Autodesk Inventor part; units mm, degrees
ref_plane "YZ Plane" through (0, 0, 0) normal (1, 0, 0) x (0, 1, 0)
ref_plane "XZ Plane" through (0, 0, 0) normal (0, 1, 0) x (-1, 0, 0)
ref_plane "XY Plane" through (0, 0, 0) normal (0, 0, 1) x (1, 0, 0)
sketch "Skizze1" plane through (0, 0, 0) normal (0, 1, 0) x (-1, 0, 0)
  line L0 (0, 25) -> (0, -25)
  line L1 (0, -25) -> (8, -25)
  line L2 (8, -25) -> (67.4432, -9.1805)
  arc A0 (67.4432, -9.1805) -> (67.4432, 9.1805) centre (65, 0) ccw
  line L3 (67.4432, 9.1805) -> (8, 25)
  line L4 (8, 25) -> (0, 25)
  line L5 (0, 0) -> (65, 0) construction
  dimension "d0" = 9.5
  dimension "d1" = 50
  dimension "d2" = 8
  dimension "d3" = 65
extrude "Extrusion1" add sketch "Skizze1" along normal blind 2
sketch "Skizze2" plane through (0, 2, 0) normal (0, 1, 0) x (1, 0, 0)
  line L0 (-67.4432, -9.1805) -> (-8, -25)
  line L1 (0, 25) -> (-8, 25)
  line L2 (-8, -25) -> (0, -25)
  line L3 (0, -25) -> (0, 25)
  line L4 (0, 25) -> (-8, 25)
  line L5 (-8, 25) -> (-8, -25)
  point P0 (0, 0)
  point P1 (-8, 25)
extrude "Extrusion2" add sketch "Skizze2" along normal blind 6.5
sketch "Skizze3" plane through (-8, 2, -25) normal (-1, 0, 0) x (0, 0, 1)
  line L0 (50, -2) -> (0, -2)
  line L1 (0, 6.5) -> (50, 6.5)
  line L2 (25, 6.5) -> (25, -12.2708) construction
  point P0 (25, -2)
  point P1 (46.124, 3)
  point P2 (3.876, 3)
  dimension "d15" = 5
  dimension "d33" = 42.248
hole "Bohrung1" at (-8, 5, 21.124) at (-8, 5, -21.124) direction (1, 0, 0) diameter 5 depth 8
sketch "Skizze4" plane through (0, 2, 0) normal (0, 1, 0) x (1, 0, 0)
  arc A0 (-67.4432, 9.1805) -> (-67.4432, -9.1805) centre (-65, 0) ccw
  point P0 (0, 0)
hole "Bohrung2" at (-65, 2, 0) direction (0, -1, 0) diameter 10 depth 2
sketch "Skizze5" plane through (0, 2, 0) normal (0, 1, 0) x (1, 0, 0)
  arc A0 (-67.4432, 9.1805) -> (-67.4432, -9.1805) centre (-65, 0) ccw
  point P0 (0, 0)
  point P1 (-51.97, 0)
  point P2 (-74.5, 0)
  dimension "d32" = 13.03
hole "Bohrung3" at (-51.97, 2, 0) direction (0, -1, 0) diameter 3.5 depth 2
properties part number "05" material "Aluminium 6061"
Build history of the part. All positions in model axes, mm. A direction names the side the tool comes from. Round coordinates to 2 decimals unless told otherwise and drop trailing zeros. Write each loop counter-clockwise with the first axis right and the second up, starting at its lowest first coordinate (ties: lowest second). Pieces come first, ordered by that corner, then holes.
1) Band-saw the part on B-B, the plane y = 5. List the corners of the cut face in (x, z), and give its area (3 significant figures).
2) Band-saw the part on D-D, the plane z = 22. List the corners of the cut face in (x, y).
3) Drill centre lines: probe 1 along X at (y, z) = (1.25, 0); probe 2 along Z at (x, y) = (-4.75, 5); probe 3 along Y at (x, z) = (-41.5, -2). Where is each one in solid material? Low to high.
4) Pin check, flat tips, straight feed: pin 1 (1 mm diameter, centred on x = -42.5, z = 3.5, fed in from -Y); pin 2 (1.5 mm diameter, centred on y = 6.5, z = -15.5, fed in from -X); pin 3 (16 mm diameter, centred on x = -65, z = 0, fed in from +Y). Stop position of each tip, or through.
5) Band-saw the part on C-C, the plane x = -65. List the corners of the cut face in (y, z), and give its area (3 significant figures).
6) Mould opens along Z. For faces 1 (the cylindrical face through (-3.94, 4.25, -18.74)), 2 (the flat face through (-8, 5, 0)), 3 (the flat face through (-37.31, 0.99, -17.2)) say: +Z half, -Z half, draft (parallel to the pull), parting line (faces both ways), or undercut.
7) 3-axis set-ups, long thin cutter, end or side, ignore diameter. For faces 4 (the flat face through (-4, 8.5, 0)), 5 (the flat face through (-33, 2, 0)): which of +Z, -Z, +X, -X, +Y, -Y reach the whole face in a straight line?
8) Band-saw the part on A-A, the plane z = 0. List the corners of the cut face in (x, y), and give its area (3 significant figures).
Ans:
1. outline: (-8, -25) - (0, -25) - (0, -23.62) - (-8, -23.62) - close; (-8, -18.62) - (0, -18.62) - (0, 18.62) - (-8, 18.62) - close; (-8, 23.62) - (0, 23.62) - (0, 25) - (-8, 25) - close
1. area: 320 mm2
2. outline: (-19.27, 0) - (0, 0) - (0, 2.66) - (-8, 2.66) - (-8, 2) - (-19.27, 2) - close; (-8, 7.34) - (0, 7.34) - (0, 8.5) - (-8, 8.5) - close
3. probe 1: x = -74.5 to -70, -60 to -53.72, -50.22 to 0
3. probe 2: z = -25 to -23.62, -18.62 to 18.62, 23.62 to 25
3. probe 3: y = 0 to 2
4. pin 1: stops at y = 0
4. pin 2: stops at x = -8
4. pin 3: stops at y = 2
5. outline: (0, -9.83) - (2, -9.83) - (2, -5) - (0, -5) - close; (0, 5) - (2, 5) - (2, 9.83) - (0, 9.83) - close
5. area: 19.3 mm2
6. face 1: undercut
6. face 2: draft
6. face 3: -Z half
7. face 4: +Z, -Z, +X, -X, +Y
7. face 5: +Z, -Z, -X, +Y
8. outline: (-74.5, 0) - (-70, 0) - (-70, 2) - (-74.5, 2) - close; (-60, 0) - (-53.72, 0) - (-53.72, 2) - (-60, 2) - close; (-50.22, 0) - (0, 0) - (0, 8.5) - (-8, 8.5) - (-8, 2) - (-50.22, 2) - close
8. area: 174 mm2
